Check sheet for the modelled part. Datum: model origin and axes. Units: mm. Face numbers are marked on the shaded views. Round coordinates to 2 decimals unless told otherwise and drop trailing zeros. Write each loop counter-clockwise with the first axis right and the second up, starting at its lowest first coordinate (ties: lowest second). Pieces come first, ordered by that corner, then holes. Notation, with made-up numbers: M -23,87 L 29,87 A20 ccw 29,109 Z; hole C 51.25,19.25 d10. An arc over 180 degrees is marked long. Put each result on its own line as item: value.
```python
from build123d import *

# Parameters (mm, degrees)
IZIM2_R                     = 5
Y_KSEKLIK_EKSTR_ZYON2_DEPTH = 30
IZIM3_R                     = 10
KES_EKSTR_ZYON1_DEPTH       = 20


with BuildPart() as part:
    # Çizim2 → Yükseklik-Ekstrüzyon2 (new body)
    with BuildSketch(Plane.XY):
        with BuildLine():
            Line((-45.944380081, 21.690872668), (4.055619919, 21.690872668))
            ThreePointArc((4.055619919, 21.690872668), (14.055619919, 11.690872668), (4.055619919, 1.690872668))
            Line((4.055619919, 1.690872668), (-45.944380081, 1.690872668))
            ThreePointArc((-45.944380081, 1.690872668), (-55.944380081, 11.690872668), (-45.944380081, 21.690872668))
        make_face()
        with Locations((-45.944380081, 11.690872668)):
            Circle(IZIM2_R, mode=Mode.SUBTRACT)
        with Locations((4.055619919, 11.690872668)):
            Circle(IZIM2_R, mode=Mode.SUBTRACT)
    extrude(amount=Y_KSEKLIK_EKSTR_ZYON2_DEPTH)

    # Çizim3 → Kes-Ekstrüzyon1 (cut)
    with BuildSketch(Plane(origin=(0, 21.690872668, 0), x_dir=(1, 0, 0), z_dir=(0, 1, 0))):
        with Locations(Location((-20.944380081, -15, 0), (0, 0, 270))):
            Circle(IZIM3_R)
    extrude(amount=-KES_EKSTR_ZYON1_DEPTH, mode=Mode.SUBTRACT)


solid = part.part
```
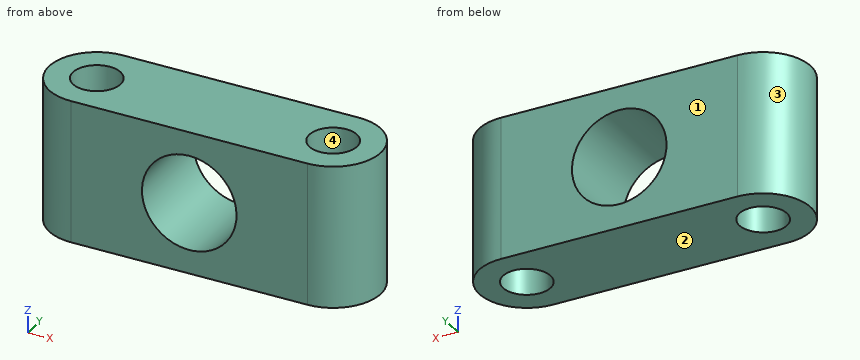
1. Depth check by flat-ended pin: pin 1 Ø6 at (y, z) = (18.5, 5) entering from -X; pin 2 Ø18 at (x, z) = (-20.94, 15) entering from +Y; pin 3 Ø6 at (y, z) = (18.5, 25.5) entering from +X; pin 4 Ø5 at (y, z) = (17, 12) entering from -X. Enter the tip coordinate at first touch or a pass-through.
Computed values:
pin 1: stops at x = -55.19
pin 2: passes through
pin 3: stops at x = 13.3
pin 4: stops at x = -55.54
2. Cross-section at A-A (z = 6.25). Enter the section's corners in (x, y), then the cut area to 3 significant figures.
Computed values:
outline: M -45.94,1.69 L -25.79,1.69 L -25.79,21.69 L -45.94,21.69 A10 ccw Z; M -16.1,1.69 L 4.06,1.69 A10 ccw 4.06,21.69 L -16.1,21.69 Z; hole C -45.94,11.69 d10; hole C 4.06,11.69 d10
area: 963 mm2
3. Cross-section at C-C (x = -20). Enter the section's corners in (y, z), then the cut area to 3 significant figures.
Computed values:
outline: M 1.69,0 L 21.69,0 L 21.69,5.04 L 1.69,5.04 Z; M 1.69,24.96 L 21.69,24.96 L 21.69,30 L 1.69,30 Z
area: 202 mm2
4. Cross-section at B-B (y = 16). Enter the section's corners in (x, z).
Computed values:
outline: M -54.97,0 L -48.48,0 L -48.48,30 L -54.97,30 Z; M -43.41,0 L 1.52,0 L 1.52,30 L -43.41,30 Z; M 6.59,0 L 13.08,0 L 13.08,30 L 6.59,30 Z; hole C -20.94,15 d20
5. Release check for a two-part mould opening along Y. For the marked faces 1, 2, 3 and 4 record: +Y half, -Y half, draft (parallel to the pull), parting line (faces both ways), or undercut.
Computed values:
face 1: +Y half
face 2: draft
face 3: parting line
face 4: undercut
6. Scan lines: probe 1 along Z at (x, y) = (-21.5, 4); probe 2 along X at (y, z) = (16, 27.5); probe 3 along X at (y, z) = (11.25, 15). Record each from-to range of solid material in increasing order.
Computed values:
probe 1: z = 0 to 5.02, 24.98 to 30
probe 2: x = -54.97 to -48.48, -43.41 to 1.52, 6.59 to 13.08
probe 3: x = -55.93 to -50.92, -40.96 to -30.94, -10.94 to -0.92, 9.04 to 14.05
7. Cross-section at D-D (z = 15). Enter the section's corners in (x, y), then the cut area to 3 significant figures.
Computed values:
outline: M -45.94,1.69 L -30.94,1.69 L -30.94,21.69 L -45.94,21.69 A10 ccw Z; M -10.94,1.69 L 4.06,1.69 A10 ccw 4.06,21.69 L -10.94,21.69 Z; hole C -45.94,11.69 d10; hole C 4.06,11.69 d10
area: 757 mm2
